```python
from build123d import *

# Parameters (mm, degrees)
SKETCH1_W           = 58.3
SKETCH1_H           = 58.3
SKETCH1_W_2         = 28.3
SKETCH1_H_2         = 28.3
BOSS_EXTRUDE1_DEPTH = 10
SKETCH4_W           = 60
SKETCH4_H           = 60
BOSS_EXTRUDE2_DEPTH = 10
SKETCH6_W           = 60
SKETCH6_H           = 26.8
ESP32_DEPTH         = 6
SKETCH8_W           = 28.3
SKETCH8_H           = 28.3
CUT_EXTRUDE3_DEPTH  = 48
SKETCH10_W          = 30
SKETCH10_H          = 5
CUT_EXTRUDE5_DEPTH  = 50
CUT_EXTRUDE2_REACH  = 95.195
SKETCH7_W           = 50
SKETCH7_H           = 3.2
CUT_EXTRUDE6_START  = -10
CUT_EXTRUDE6_DEPTH  = 71.932070392
CUT_EXTRUDE7_START  = -25
CUT_EXTRUDE7_DEPTH  = 50
CUT_EXTRUDE8_REACH  = 102.747
SKETCH14_W          = 15
SKETCH14_H          = 3
CUT_EXTRUDE9_DEPTH  = 48
CHAMFER1_SIZE       = 7.5
CUT_EXTRUDE10_REACH = 81.712
SKETCH15_R          = 2.65
SKETCH16_W          = 15.4
SKETCH16_H          = 16.6
CANBUS_DEPTH        = 3
SKETCH18_R          = 1.05
M2_CANBUS_DEPTH     = 6
SKETCH19_R          = 2.75
CUT_EXTRUDE13_DEPTH = 8
SKETCH20_R          = 2.75
CUT_EXTRUDE14_DEPTH = 8
SKETCH21_R          = 2.75
CUT_EXTRUDE15_DEPTH = 8
CUT_EXTRUDE16_START = -8
SKETCH22_R          = 2.75
CUT_EXTRUDE16_DEPTH = 8


# Read off the part's stored shape, not the designer's step: Cut-Extrude7
with BuildPart() as part:
    # Sketch1 → Boss-Extrude1 (new body)
    # profile 1 of 2: a face of its own
    with BuildSketch(Plane(origin=(0, 0, 0), x_dir=(1, 0, 0), z_dir=(0, 1, 0))):
        Rectangle(SKETCH1_W, SKETCH1_H)
        Rectangle(SKETCH1_W_2, SKETCH1_H_2, mode=Mode.SUBTRACT)
    # profile 2 of 2: a face of its own
    with BuildSketch(Plane(origin=(0, 0, 0), x_dir=(1, 0, 0), z_dir=(0, 1, 0))):
        Rectangle(SKETCH1_W_2, SKETCH1_H_2)
    extrude(amount=BOSS_EXTRUDE1_DEPTH)

    # Sketch2 → section 1 of loft1
    with BuildSketch(Plane(origin=(0, 40, 0), x_dir=(1, 0, 0), z_dir=(0, 1, 0)), mode=Mode.PRIVATE) as loft1_s1:
        with BuildLine():
            Line((-45, -45), (45, -45))
            Line((45, -45), (45, 45))
            Line((45, 45), (-45, 45))
            Line((-45, 45), (-45, -45))
        make_face()
    # loft from a face of the part (loft1)
    loft([part.faces().sort_by_distance((0, 10, 0))[0], loft1_s1.sketch])

    # Sketch4 → Boss-Extrude2 (add)
    with BuildSketch(Plane(origin=(0, 40, 0), x_dir=(1, 0, 0), z_dir=(0, 1, 0))):
        Rectangle(SKETCH4_W, SKETCH4_H)
    extrude(amount=BOSS_EXTRUDE2_DEPTH)

    # Sketch6 → ESP32 (cut)
    with BuildSketch(Plane(origin=(0, -9.857868483, -18.658426151), x_dir=(-1, 0, 0), z_dir=(0, -0.4671427704257183, -0.8841818998594039))):
        with Locations((0, 37.859030757)):
            Rectangle(SKETCH6_W, SKETCH6_H)
    extrude(amount=-ESP32_DEPTH, mode=Mode.SUBTRACT)

    # Sketch8 → Cut-Extrude3 (cut)
    with BuildSketch(Plane(origin=(0, 50, 0), x_dir=(1, 0, 0), z_dir=(0, 1, 0))):
        Rectangle(SKETCH8_W, SKETCH8_H)
    extrude(amount=-CUT_EXTRUDE3_DEPTH, mode=Mode.SUBTRACT)

    # Sketch10 → Cut-Extrude5 (cut)
    with BuildSketch(Plane(origin=(0, 0, 0), x_dir=(-1, 0, 0), z_dir=(0, -1, 0))):
        with Locations((0, 19.65)):
            Rectangle(SKETCH10_W, SKETCH10_H)
    extrude(amount=-CUT_EXTRUDE5_DEPTH, mode=Mode.SUBTRACT)

    # Cut-Extrude2: up to this plane
    cut_extrude2_end = Plane(origin=(-15, 50, -22.15), z_dir=(0, 0, -1))
    # Sketch7 → Cut-Extrude2 (cut, up to the surface)
    with BuildSketch(Plane(origin=(0, -7.055011861, -13.353334752), x_dir=(-1, 0, 0), z_dir=(0, -0.46714277042571845, -0.8841818998594037)), mode=Mode.PRIVATE) as cut_extrude2_sk1:
        with Locations((0, 47.659030757)):
            Rectangle(SKETCH7_W, SKETCH7_H)
    cut_extrude2_tool1 = split(extrude(cut_extrude2_sk1.sketch, amount=-CUT_EXTRUDE2_REACH, mode=Mode.PRIVATE), bisect_by=cut_extrude2_end, keep=Keep.BOTH, mode=Mode.PRIVATE)
    add(cut_extrude2_tool1.solids().sort_by_distance((0, 35.08424, -35.616906))[0], mode=Mode.SUBTRACT)
    # Sketch7 → Cut-Extrude2 (cut, up to the surface)
    with BuildSketch(Plane(origin=(0, -7.055011861, -13.353334752), x_dir=(-1, 0, 0), z_dir=(0, -0.46714277042571845, -0.8841818998594037)), mode=Mode.PRIVATE) as cut_extrude2_sk2:
        with Locations((0, 28.059030757)):
            Rectangle(SKETCH7_W, SKETCH7_H)
    cut_extrude2_tool2 = split(extrude(cut_extrude2_sk2.sketch, amount=-CUT_EXTRUDE2_REACH, mode=Mode.PRIVATE), bisect_by=cut_extrude2_end, keep=Keep.BOTH, mode=Mode.PRIVATE)
    add(cut_extrude2_tool2.solids().sort_by_distance((0, 17.754275, -26.460908))[0], mode=Mode.SUBTRACT)

    # Sketch11 → Cut-Extrude6 (cut, through all)
    with BuildSketch(Plane(origin=(0, 50, 0), x_dir=(1, 0, 0), z_dir=(0, 1, 0)).offset(CUT_EXTRUDE6_START)):
        Polygon((-25, 22.15), (25, 22.15), (15, 17.15), (-15, 17.15), align=None)
    extrude(amount=-CUT_EXTRUDE6_DEPTH, mode=Mode.SUBTRACT)

    # Cut-Extrude7 outline → Cut-Extrude7 (cut)
    with BuildSketch(Plane.YZ.offset(CUT_EXTRUDE7_START)):
        Polygon((40.38967366, -22.15), (21.841454111, -22.15), (21.504680154, -22.787427049), (36.005263311, -30.448568484), align=None)
    extrude(amount=CUT_EXTRUDE7_DEPTH, mode=Mode.SUBTRACT)

    # Cut-Extrude8: up to this plane
    cut_extrude8_end = Plane(origin=(18.658426151, -9.857868483, 0), z_dir=(-0.884181899859404, 0.4671427704257181, 0))
    # Sketch13 → Cut-Extrude8 (cut, up to the surface)
    with BuildSketch(Plane.ZY.offset(-30), mode=Mode.PRIVATE) as cut_extrude8_sk1:
        Polygon((-32.139713731, 15.658764159), (-40.548283598, 31.574038357), (-35.243192199, 34.376894979), (-26.834622332, 18.461620782), align=None)
    cut_extrude8_tool1 = split(extrude(cut_extrude8_sk1.sketch, amount=-CUT_EXTRUDE8_REACH, mode=Mode.PRIVATE), bisect_by=cut_extrude8_end, keep=Keep.BOTH, mode=Mode.PRIVATE)
    add(cut_extrude8_tool1.solids().sort_by_distance((30, 25.01783, -33.691453))[0], mode=Mode.SUBTRACT)

    # Sketch14 → Cut-Extrude9 (cut)
    with BuildSketch(Plane(origin=(0, 50, 0), x_dir=(1, 0, 0), z_dir=(0, 1, 0))):
        with Locations((0, 15.65)):
            Rectangle(SKETCH14_W, SKETCH14_H)
    extrude(amount=-CUT_EXTRUDE9_DEPTH, mode=Mode.SUBTRACT)

    # Chamfer1
    # the kernel refuses this chamfer: 7.5 mm, written as the material it adds along each edge
    with BuildSketch(Plane(origin=(15, 40, -17.15), x_dir=(-0.9996219169112968, 0, 0.02749587661058632), z_dir=(0, 1, 0))) as chamfer1_piece_1_section:
        Polygon((CHAMFER1_SIZE * 0.999621916911, -CHAMFER1_SIZE * 0.0274958766106), (-CHAMFER1_SIZE * 0.0274958766106, -CHAMFER1_SIZE * 0.999621916911), (0, 0), align=None)
    chamfer1_piece_1 = extrude(amount=10, mode=Mode.PRIVATE)
    chamfer1_piece_1 = split(chamfer1_piece_1, bisect_by=Plane(origin=(12.200765376, 42.822931518, -22.15), z_dir=(0, 0, 1)), keep=Keep.TOP, mode=Mode.PRIVATE)
    add(chamfer1_piece_1)
    with BuildSketch(Plane(origin=(-15, 40, -17.15), x_dir=(0.9996219169112968, 0, 0.02749587661058632), z_dir=(0, 1, 0))) as chamfer1_piece_2_section:
        Polygon((CHAMFER1_SIZE * 0.999621916911, CHAMFER1_SIZE * 0.0274958766106), (-CHAMFER1_SIZE * 0.0274958766106, CHAMFER1_SIZE * 0.999621916911), (0, 0), align=None)
    chamfer1_piece_2 = extrude(amount=10, mode=Mode.PRIVATE)
    chamfer1_piece_2 = split(chamfer1_piece_2, bisect_by=Plane(origin=(-12.200765376, 42.822931518, -22.15), z_dir=(0, 0, 1)), keep=Keep.TOP, mode=Mode.PRIVATE)
    add(chamfer1_piece_2)

    # Sketch15 → Cut-Extrude10 (cut, up to next)
    with BuildSketch(Plane(origin=(0, 2, 0), x_dir=(1, 0, 0), z_dir=(0, 1, 0)), mode=Mode.PRIVATE) as cut_extrude10_sk1:
        with Locations(Location((0, 0, 0), (0, 0, 270))):
            Circle(SKETCH15_R)
    cut_extrude10_tool1 = extrude(cut_extrude10_sk1.sketch, amount=-CUT_EXTRUDE10_REACH, mode=Mode.PRIVATE) & part.part
    add(cut_extrude10_tool1.solids().sort_by_distance((0, 2, 0))[0], mode=Mode.SUBTRACT)

    # Sketch16 → CANbus (cut)
    with BuildSketch(Plane(origin=(-18.658426151, -9.857868483, 0), x_dir=(0, 0, 1), z_dir=(-0.8841818998594037, -0.46714277042571845, 0))):
        with Locations((0, 40.759030757)):
            Rectangle(SKETCH16_W, SKETCH16_H)
    extrude(amount=-CANBUS_DEPTH, mode=Mode.SUBTRACT)

    # Sketch18 → M2-CANbus (cut)
    with BuildSketch(Plane(origin=(-16.005880452, -8.456440172, 0), x_dir=(0, 0, 1), z_dir=(-0.8841818998594035, -0.46714277042571867, 0))):
        with Locations(Location((5.2, 45.898343703, 0), (0, 0, 270))):
            Circle(SKETCH18_R)
        with Locations(Location((5.2, 34.898343703, 0), (0, 0, 270))):
            Circle(SKETCH18_R)
    extrude(amount=-M2_CANBUS_DEPTH, mode=Mode.SUBTRACT)

    # Sketch19 → Cut-Extrude13 (cut)
    with BuildSketch(Plane(origin=(0, 0, -30), x_dir=(-1, 0, 0), z_dir=(0, 0, -1))):
        with Locations((-22.5, 45)):
            Circle(SKETCH19_R)
        with Locations((22.5, 45)):
            Circle(SKETCH19_R)
    extrude(amount=-CUT_EXTRUDE13_DEPTH, mode=Mode.SUBTRACT)

    # Sketch20 → Cut-Extrude14 (cut)
    with BuildSketch(Plane(origin=(30, 0, 0), x_dir=(0, 0, -1), z_dir=(1, 0, 0))):
        with Locations((0, 45)):
            Circle(SKETCH20_R)
    extrude(amount=-CUT_EXTRUDE14_DEPTH, mode=Mode.SUBTRACT)

    # Sketch21 → Cut-Extrude15 (cut)
    with BuildSketch(Plane.XY.offset(30)):
        with Locations((0, 45)):
            Circle(SKETCH21_R)
    extrude(amount=-CUT_EXTRUDE15_DEPTH, mode=Mode.SUBTRACT)

    # Sketch22 → Cut-Extrude16 (cut)
    with BuildSketch(Plane.ZY.offset(30).offset(CUT_EXTRUDE16_START)):
        with Locations(Location((0, 45, 0), (0, 0, 180))):
            Circle(SKETCH22_R)
    extrude(amount=CUT_EXTRUDE16_DEPTH, mode=Mode.SUBTRACT)


solid = part.part
```
Input: part model. Units: mm. Frame: model coordinates. A direction names the side the tool comes from. Coordinates: 2 decimals unless noted, no trailing zeros. Use a Markdown table: item, result.
1) Pull-direction query (X, two-part tool) for faces 1 (the flat face through (31.38, 17.08, -29.45)), 2 (the flat face through (-30, 25, -34)), 3 (the flat face through (-0.35, 28.653, -26.564)), 4 (the flat face through (29.15, 5, 0)); classes: released by +X, released by -X, zero draft, split by the parting line, or undercut.
Results found:
| item | result |
|---|---|
| face 1 | zero draft |
| face 2 | undercut |
| face 3 | undercut |
| face 4 | released by +X |
2) Access query for faces 5 (the flat face through (23, 45, -22)), 6 (the flat face through (0.35, 34.82, -32.69)), 7 (the flat face through (0, 5, 29.15)). Directions: +Z, -Z, +X, -X, +Y, -Y. A direction counts if a zero-diameter tool reaches every point of the face in a straight line with its end or side. Return the directions, or none.
Results found:
| item | result |
|---|---|
| face 5 | -Z |
| face 6 | none |
| face 7 | +Z, +X, -X, -Y |
3) Contact query for flat-ended pins moving along their axis: pin 1 (14.5 mm diameter, centred on y = 26, z = -31.5, fed in from +X); pin 2 (11 mm diameter, centred on y = 5, z = -0.5, fed in from +X); pin 3 (9 mm diameter, centred on x = -22.5, y = 45, fed in from -Z); pin 4 (3 mm diameter, centred on x = -22.5, z = 23, fed in from -Y). Output: stop coordinate, or through.
Results found:
| item | result |
|---|---|
| pin 1 | stops at x = 41.43 |
| pin 2 | stops at x = 29.41 |
| pin 3 | stops at z = -30 |
| pin 4 | stops at y = 0 |
4) Cut plane A-A (x = 0). Give the number of separate pieces and of enclosed holes in the cut face, then the cut area to 3 significant figures.
Results found:
| item | result |
|---|---|
| separate pieces | 5 |
| enclosed holes | 0 |
| area | 1,290 mm2 |
5) Material intervals for line 1 along Y through (x, z) = (22.5, -26.5); line 2 along Z through (x, y) = (-28, 45); line 3 along Y through (x, z) = (-24.25, 0), sorted ascending. Write a range as from..to.
Results found:
| item | result |
|---|---|
| line 1 | y = 0..13.66, 19.54..28.53, 41.71..42.25, 47.75..50 |
| line 2 | z = -30..-2.75, 2.75..30 |
| line 3 | y = 0..42.25, 47.75..50 |
